from build123d import *

# Parameters (mm, degrees)
BOSS_EXTRUDE1_DEPTH      = 19.05
SHELL3_START             = -16.51
SHELL3_DEPTH             = 35.56
SKETCH7_W                = 9.144
SKETCH7_H                = 21.336
SKETCH7_R                = 3.302
BOSS_EXTRUDE3_DEPTH      = 12.7
CHAMFER1_SIZE            = 15.24
CHAMFER1_SIZE_2          = 7.62
CUT_EXTRUDE4_DEPTH       = 13.335
BOSS_EXTRUDE4_DEPTH      = 1.27
BOSS_EXTRUDE4_DEPTH_BACK = 12.7
SKETCH9_R                = 3.175
CUT_EXTRUDE5_DEPTH       = 2.54
FILLET1_R                = 2.54
FILLET2_R                = 2.54


# Read off the part's stored shape, not the designer's step: Shell3
with BuildPart() as part:
    # Sketch1 → Boss-Extrude1 (new, symmetric)
    with BuildSketch(Plane.XY):
        with BuildLine():
            Line((-57.15, -31.75), (57.15, -31.75))
            Line((57.15, -31.75), (57.15, 31.75))
            Line((57.15, 31.75), (-49.022, 31.75))
            Line((-49.022, 31.75), (-49.022, 42.144910037))
            Line((-49.022, 42.144910037), (-51.100806987, 42.144910037))
            Line((-51.100806987, 42.144910037), (-66.686518268, 47.249120101))
            Line((-66.686518268, 47.249120101), (-66.686518268, 49.174694101))
            ThreePointArc((-66.686518268, 49.174694101), (-68.789611639, 54.223594812), (-73.855077994, 56.286469196))
            Line((-73.855077994, 56.286469196), (-73.968197446, 56.286469196))
            ThreePointArc((-73.968197446, 56.286469196), (-78.960538431, 54.18360073), (-81.02363772, 49.174694101))
            Line((-81.02363772, 49.174694101), (-81.02363772, 47.249120101))
            ThreePointArc((-81.02363772, 47.249120101), (-93.341814168, 31.674687064), (-81.02363772, 16.100254027))
            Line((-81.02363772, 16.100254027), (-81.02363772, 14.174680027))
            ThreePointArc((-81.02363772, 14.174680027), (-78.940581148, 9.145736599), (-73.91163772, 7.062680027))
            Line((-73.91163772, 7.062680027), (-73.798518268, 7.062680027))
            ThreePointArc((-73.798518268, 7.062680027), (-68.74596031, 9.210475671), (-66.728346573, 14.31641367))
            Line((-66.728346573, 14.31641367), (-66.687998915, 16.24156491))
            Line((-66.687998915, 16.24156491), (-57.15, 16.24156491))
            Line((-57.15, 16.24156491), (-57.15, -31.75))
        make_face()
    extrude(amount=BOSS_EXTRUDE1_DEPTH, both=True)

    # Shell3 outline → Shell3 (cut)
    with BuildSketch(Plane.XY.offset(SHELL3_START)):
        with BuildLine():
            Line((54.61, 29.21), (-51.562, 29.21))
            Line((-51.562, 29.21), (-51.562, 39.623206475))
            Line((-51.562, 39.623206475), (-69.226518268, 45.408211104))
            Line((-69.226518268, 45.408211104), (-69.226518268, 49.174694101))
            ThreePointArc((-69.226518268, 49.174694101), (-70.581699125, 52.423579848), (-73.843866737, 53.746469196))
            Line((-73.843866737, 53.746469196), (-73.956986189, 53.746469196))
            ThreePointArc((-73.956986189, 53.746469196), (-77.160523467, 52.391513244), (-78.48363772, 49.174694101))
            Line((-78.48363772, 49.174694101), (-78.48363772, 45.090596577))
            ThreePointArc((-78.48363772, 45.090596577), (-90.801814168, 31.674687064), (-78.48363772, 18.258777551))
            Line((-78.48363772, 18.258777551), (-78.48363772, 14.174680027))
            ThreePointArc((-78.48363772, 14.174680027), (-77.144529924, 10.941787823), (-73.91163772, 9.602680027))
            Line((-73.91163772, 9.602680027), (-73.806528971, 9.602680027))
            ThreePointArc((-73.806528971, 9.602680027), (-70.546554352, 11.002273539), (-69.268997314, 14.311978137))
            Line((-69.268997314, 14.311978137), (-69.175322928, 18.78156491))
            Line((-69.175322928, 18.78156491), (-54.61, 18.78156491))
            Line((-54.61, 18.78156491), (-54.61, -29.21))
            Line((-54.61, -29.21), (54.61, -29.21))
            Line((54.61, -29.21), (54.61, 29.21))
        make_face()
    extrude(amount=SHELL3_DEPTH, mode=Mode.SUBTRACT)

    # Sketch7 → Boss-Extrude3 (add)
    with BuildSketch(Plane(origin=(0, 31.75, 0), x_dir=(1, 0, 0), z_dir=(0, 1, 0))):
        with Locations((50.8, -17.018)):
            Rectangle(SKETCH7_W, SKETCH7_H)
        with Locations(Location((50.8, -22.606, 0), (0, 0, 180))):
            Circle(SKETCH7_R, mode=Mode.SUBTRACT)
    extrude(amount=BOSS_EXTRUDE3_DEPTH)

    # Chamfer1
    # the kernel refuses this chamfer: 15.24, 7.62 mm, written as the material it takes off along each edge
    with BuildSketch(Plane(origin=(57.15, -71.218992037, 19.05), x_dir=(-0.9998508956747117, 0, 0.017268075123668167), z_dir=(0, 1, 0))) as chamfer1_piece_1:
        Polygon((CHAMFER1_SIZE * 0.999850895675, -CHAMFER1_SIZE * 0.0172680751237), (-CHAMFER1_SIZE_2 * 0.0172680751237, -CHAMFER1_SIZE_2 * 0.999850895675), (0, 0), align=None)
    extrude(amount=102.968992037, mode=Mode.SUBTRACT)

    # Sketch8 → Cut-Extrude4 (cut)
    with BuildSketch(Plane.XY.offset(19.05)):
        with BuildLine():
            Line((-66.610527579, 49.002799892), (-66.610527579, 47.279305102))
            Line((-66.610527579, 47.279305102), (-51.100806987, 42.144910037))
            Line((-51.100806987, 42.144910037), (-38.403655113, 42.144910037))
            Line((-38.403655113, 42.144910037), (-38.403655113, 16.24156491))
            Line((-38.403655113, 16.24156491), (-66.687998915, 16.24156491))
            Line((-66.687998915, 16.24156491), (-66.726931852, 14.174565202))
            ThreePointArc((-66.726931852, 14.174565202), (-67.907528646, 10.164808506), (-71.108849398, 7.477150977))
            ThreePointArc((-71.108849398, 7.477150977), (-77.894512097, 8.119410548), (-81.02363772, 14.174680027))
            Line((-81.02363772, 14.174680027), (-81.02363772, 16.100254027))
            ThreePointArc((-81.02363772, 16.100254027), (-93.341814168, 31.674687064), (-81.02363772, 47.249120101))
            Line((-81.02363772, 47.249120101), (-81.02363772, 49.174694101))
            ThreePointArc((-81.02363772, 49.174694101), (-80.441084846, 51.993712411), (-78.788861502, 54.350912042))
            ThreePointArc((-78.788861502, 54.350912042), (-70.907499507, 55.757912789), (-66.610527579, 49.002799892))
        make_face()
    extrude(amount=-CUT_EXTRUDE4_DEPTH, mode=Mode.SUBTRACT)

    # Sketch9 → Boss-Extrude4 (add, two sides: drawn at the far end of the back side and taken through both)
    with BuildSketch(Plane(origin=(-93.341814168, 0, 0), x_dir=(0, 0, -1), z_dir=(1, 0, 0)).offset(-BOSS_EXTRUDE4_DEPTH_BACK)):
        with Locations(Location((-1.905, 31.75, 0), (0, 0, 90))):
            Circle(SKETCH9_R)
    extrude(amount=BOSS_EXTRUDE4_DEPTH + BOSS_EXTRUDE4_DEPTH_BACK)

    # Sketch10 → Cut-Extrude5 (cut)
    with BuildSketch(Plane(origin=(57.15, 0, 0), x_dir=(0, 0, -1), z_dir=(1, 0, 0))):
        Polygon((-19.05, -29.21), (-13.314117838, -29.21), (-13.314117838, -22.878143144), (-3.81, -22.878143144), (-3.81, -10.729059706), (-13.314117838, -10.729059706), (-13.314117838, 3.974723841), (-3.81, 3.974723841), (-3.81, 19.366104348), (-13.314117838, 19.366104348), (-13.314117838, 29.21), (-19.05, 29.21), align=None)
    extrude(amount=-CUT_EXTRUDE5_DEPTH, mode=Mode.SUBTRACT)

    # Fillet1
    fillet1_edges = [part.edges().sort_by_distance(p)[0] for p in [
        (-81.02363772, 16.100254027, -6.6675),
        (-78.48363772, 18.258777551, -5.3975),
        (-69.175322928, 18.78156491, -5.3975),
        (-66.687998915, 16.24156491, -6.6675),
        (-69.226518268, 45.408211104, -5.3975),
        (-66.686518268, 47.249120101, -6.6675),
        (-81.02363772, 47.249120101, -6.6675),
        (-78.48363772, 45.090596577, -5.3975),
    ]]
    fillet(fillet1_edges, radius=FILLET1_R)

    # Fillet2
    fillet2_edges = [part.edges().sort_by_distance(p)[0] for p in [
        (41.91, 30.48, 19.05),
        (41.91, -30.48, 19.05),
    ]]
    fillet(fillet2_edges, radius=FILLET2_R)


solid = part.part
Input: part model. Units: mm. Frame: model coordinates. A direction names the side the tool comes from. Give positions to 0.01 mm unless a question says otherwise; leave off trailing zeros. Loops run counter-clockwise (first coordinate to the right, second up) from the corner with the lowest first, then second, coordinate; pieces in that order, holes last. Notation, with made-up numbers: (43, 22) -> (75, 22) arc R25 cw to (75, 49) -> close; hole circle Ø9 at (21.25, 73.25). An arc over 180 degrees is marked (long way). Answer as a JSON object with one key per item and string values. Group by question number.
Item 1: Line query: probe 1 along Z at (x, y) = (50.8, 39); probe 2 along X at (y, z) = (-14, -11.5); probe 3 along Y at (x, z) = (-26, -4). Output: solid intervals per line, ascending.
Item 2: Reachability of faces 4 (the flat face through (51, 38, 6.35)), 5 (the flat face through (51.398, 29.657, 14.306)), 6 (the flat face through (-19, 4, -16.51)) from +Z, -Z, +X, -X, +Y, -Y: full face, straight path, thin tool, end or side. Return the list, or none.
Item 3: Pin query (flat end, axial travel): P1, Ø3, axis at x = 8.5, y = 30.5, coming from the +Z side; P2, Ø5, axis at x = -28, y = 5.5, coming from the +Z side; P3, Ø7.5, axis at x = 51, z = 20, coming from the -Y side. Return the tip coordinate at first contact, or that it passes through.
Item 4: Cut plane B-B, the plane x = 50.8. Return the cut outline in (y, z) (3 decimals), and give its area (3 significant figures).
Item 5: Pull-direction query (X, two-part tool) for faces 1 (the flat face through (-106.042, 32, 2)), 2 (the cylindrical face through (-99.616, 31.062, -1.194)), 3 (the flat face through (-59.408, 42.193, -5.553)); classes: released by +X, released by -X, zero draft, split by the parting line, or undercut.
Item 6: Cut plane A-A, the plane y = -6. Return the cut outline in (x, z).
Item 7: Cut plane C-C, the plane x = -59. Return the cut outline in (y, z) (3 decimals).
Checks:
{
 "1": {"probe 1": "z = 6.35 to 19.3, 25.91 to 27.69", "probe 2": "x = -57.15 to -54.61, 54.61 to 57.15", "probe 3": "y = -31.75 to -29.21, 29.21 to 31.75"},
 "2": {"face 4": "-Z, +X, -X, +Y", "face 5": "+Z, +X, -Y", "face 6": "+Z"},
 "3": {"P1": "stops at z = 19.05", "P2": "stops at z = -16.51", "P3": "stops at y = 31.75"},
 "4": {"outline": "(-31.75, -19.05) -> (31.75, -19.05) -> (31.75, 6.35) -> (44.45, 6.35) -> (44.45, 19.304) -> (31.75, 19.304) -> (31.75, 14.605) -> (29.21, 14.605) -> (29.21, -16.51) -> (-29.21, -16.51) -> (-29.21, 14.605) -> (-31.75, 14.605) -> close; (31.75, 25.908) -> (44.45, 25.908) -> (44.45, 27.686) -> (31.75, 27.686) -> close", "area": "506 mm²"},
 "5": {"face 1": "released by -X", "face 2": "zero draft", "face 3": "undercut"},
 "6": {"outline": "(-57.15, -19.05) -> (57.15, -19.05) -> (57.15, 11.43) -> (54.61, 12.7) -> (54.61, -16.51) -> (-54.61, -16.51) -> (-54.61, 19.05) -> (-57.15, 19.05) -> close"},
 "7": {"outline": "(16.242, -19.05) -> (44.732, -19.05) -> (44.732, 5.715) -> (42.059, 5.715) -> (42.059, -16.51) -> (18.782, -16.51) -> (18.782, 5.715) -> (16.242, 5.715) -> close"}
}
